from build123d import *

# Parameters (mm, degrees)
SKETCH1_W          = 25.4
SKETCH1_H          = 228.6
EXTRUDE1_DEPTH     = 3.175
SKETCH3_W          = 3.175
SKETCH3_H          = 6.35
CUT_EXTRUDE1_DEPTH = 3.175
LPATTERN1_COUNT    = 2
LPATTERN1_PITCH    = 222.25
SKETCH4_W          = 3.175
SKETCH4_H          = 12.7
CUT_EXTRUDE2_DEPTH = 3.175
LPATTERN2_COUNT    = 8
LPATTERN2_PITCH    = 25.4
SKETCH5_W          = 12.7
SKETCH5_H          = 3.175
CUT_EXTRUDE3_DEPTH = 3.175
SKETCH6_W          = 6.35
SKETCH6_H          = 3.175
CUT_EXTRUDE4_DEPTH = 3.175
LPATTERN3_COUNT    = 2
LPATTERN3_PITCH    = 19.05


with BuildPart() as part:
    # Sketch1 → Extrude1 (new body)
    with BuildSketch(Plane.XY):
        with Locations((12.7, 114.3)):
            Rectangle(SKETCH1_W, SKETCH1_H)
    extrude(amount=EXTRUDE1_DEPTH)

    # Sketch3 → Cut-Extrude1 (cut)
    with BuildSketch(Plane.XY.offset(3.175)):
        with Locations((23.8125, 225.425)):
            Rectangle(SKETCH3_W, SKETCH3_H)
    cut_extrude1 = extrude(amount=-CUT_EXTRUDE1_DEPTH, mode=Mode.SUBTRACT)

    # LPattern1: Cut-Extrude1 ×2
    with Locations(*[(0, -i * LPATTERN1_PITCH, 0) for i in range(1, LPATTERN1_COUNT)]):
        add(cut_extrude1, mode=Mode.SUBTRACT)

    # Sketch4 → Cut-Extrude2 (cut)
    with BuildSketch(Plane.XY.offset(3.175)):
        with Locations((23.8125, 203.2)):
            Rectangle(SKETCH4_W, SKETCH4_H)
    cut_extrude2 = extrude(amount=-CUT_EXTRUDE2_DEPTH, mode=Mode.SUBTRACT)

    # LPattern2: Cut-Extrude2 ×8
    with Locations(*[(0, -i * LPATTERN2_PITCH, 0) for i in range(1, LPATTERN2_COUNT)]):
        add(cut_extrude2, mode=Mode.SUBTRACT)

    # Sketch5 → Cut-Extrude3 (cut)
    with BuildSketch(Plane.XY.offset(3.175)):
        with Locations((12.7, 1.5875)):
            Rectangle(SKETCH5_W, SKETCH5_H)
    extrude(amount=-CUT_EXTRUDE3_DEPTH, mode=Mode.SUBTRACT)

    # Sketch6 → Cut-Extrude4 (cut)
    with BuildSketch(Plane.XY.offset(3.175)):
        with Locations((3.175, 227.0125)):
            Rectangle(SKETCH6_W, SKETCH6_H)
    cut_extrude4 = extrude(amount=-CUT_EXTRUDE4_DEPTH, mode=Mode.SUBTRACT)

    # LPattern3: Cut-Extrude4 ×2
    with Locations(*[(i * LPATTERN3_PITCH, 0, 0) for i in range(1, LPATTERN3_COUNT)]):
        add(cut_extrude4, mode=Mode.SUBTRACT)


solid = part.part
Geometry: final body of the model. Coordinates: model frame, mm. Round coordinates to 2 decimals unless told otherwise and drop trailing zeros. Order: outer loops, then holes, each group sorted by start corner. A loop starts at its lowest first (then second) coordinate and runs counter-clockwise, first axis right, second up.
Q1. Pin query (flat end, axial travel): pin 1 (1.6 mm diameter, centred on y = 1, z = 1, fed in from +X) (3 decimals); pin 2 (1 mm diameter, centred on x = 17, z = 2.5, fed in from -Y) (3 decimals); pin 3 (1 mm diameter, centred on x = 23.5, z = 2, fed in from -Y). Return the tip coordinate at first contact, or that it passes through.
Result sheet:
pin 1: stops at x = 22.225
pin 2: stops at y = 3.175
pin 3: stops at y = 6.35
Q2. Material intervals for probe 1 along Y at (x, z) = (18, 1.25) (3 decimals); probe 2 along Y at (x, z) = (1.5, 0.85) (3 decimals); probe 3 along X at (y, z) = (205, 1.65) (3 decimals), sorted ascending.
Result sheet:
probe 1: y = 3.175 to 228.6
probe 2: y = 0 to 225.425
probe 3: x = 0 to 22.225
Q3. Section A-A, the plane y = 181. Output: boundary loops of the cut face in (x, z) (3 decimals).
Result sheet:
outline: (0, 0) - (22.225, 0) - (22.225, 3.175) - (0, 3.175) - close
